Read the model definition and answer for the solid it produces. Units are mm, in the model's axes. Coordinates: 2 decimals unless noted, no trailing zeros. Order: outer loops, then holes, each group sorted by start corner. A loop starts at its lowest first (then second) coordinate and runs counter-clockwise, first axis right, second up. Notation, with made-up numbers: (66.25, -12.5) -> (117.25, -12.5) arc R8 cw to (117.25, -2.5) -> close; hole circle Ø2 at (-31.75, 35). An arc over 180 degrees is marked (long way). Answer as a JSON object with one key per item and string values. Group by question number.
1) Given pin 1 (1.5 mm diameter, centred on x = -0.5, y = 1.5, fed in from -Z); pin 2 (0.8 mm diameter, centred on x = -8, y = 1, fed in from +Z); pin 3 (0.8 mm diameter, centred on y = 1.5, z = 8, fed in from +X), each flat-ended and moving along its own axis, determine where each tip first touches the part or whether it passes through.
2) Section C-C on y = 2.5 is taken. Determine the outline of the cut face in (x, z), and give its area (3 significant figures).
3) Section B-B on x = 0 is taken. Determine the outline of the cut face in (y, z), and give its area (3 significant figures).
4) Determine the mould class of faces 1 (the cylindrical face through (9.7, 1.48, 6.18)), 2 (the flat face through (-3, 1, -8)), 3 (the flat face through (-2, 0, 0)) for opening direction Z: released by +Z, released by -Z, zero draft, split by the parting line, or undercut.
5) Section D-D on z = 7.5 is taken. Determine the outline of the cut face in (x, y), and give its area (3 significant figures).
6) Consider L1, parallel to X at y = 0.85, z = 0; L2, parallel to X at y = 2.15, z = 2.5; L3, parallel to Z at x = 2.25, y = 2.2. Determine where each line is inside the solid, lowest interval first.
7) Section A-A on z = 0 is taken. Determine the outline of the cut face in (x, y), and give its area (3 significant figures).
from build123d import *

# Parameters (mm, degrees)
SKETCH5_R           = 11.5
BOSS_EXTRUDE2_DEPTH = 3
SKETCH3_W           = 6
SKETCH3_H           = 2.5
SKETCH3_W_2         = 2.5
SKETCH3_H_2         = 6
CUT_EXTRUDE1_DEPTH  = 3
SKETCH6_R           = 1.35
CUT_EXTRUDE2_DEPTH  = 3


with BuildPart() as part:
    # Sketch5 → Boss-Extrude2 (new body)
    with BuildSketch(Plane(origin=(0, 0, 0), x_dir=(1, 0, 0), z_dir=(0, 1, 0))):
        with Locations(Location((0, 0, 0), (0, 0, 270))):
            Circle(SKETCH5_R)
    extrude(amount=BOSS_EXTRUDE2_DEPTH)

    # Sketch3 → Cut-Extrude1 (cut)
    with BuildSketch(Plane(origin=(0, 0, 0), x_dir=(1, 0, 0), z_dir=(0, 1, 0))):
        with Locations((0, 7.75)):
            Rectangle(SKETCH3_W, SKETCH3_H)
        with Locations((7.75, 0)):
            Rectangle(SKETCH3_W_2, SKETCH3_H_2)
        with Locations((0, -7.75)):
            Rectangle(SKETCH3_W, SKETCH3_H)
        with Locations((-7.75, 0)):
            Rectangle(SKETCH3_W_2, SKETCH3_H_2)
    extrude(amount=CUT_EXTRUDE1_DEPTH, mode=Mode.SUBTRACT)

    # Sketch6 → Cut-Extrude2 (cut)
    with BuildSketch(Plane(origin=(0, 3, 0), x_dir=(1, 0, 0), z_dir=(0, 1, 0))):
        with Locations(Location((0, 0, 0), (0, 0, 270))):
            Circle(SKETCH6_R)
    extrude(amount=-CUT_EXTRUDE2_DEPTH, mode=Mode.SUBTRACT)


solid = part.part
Worked answers:
{
 "1": {"pin 1": "stops at z = -11.5", "pin 2": "stops at z = 8.63", "pin 3": "stops at x = 8.63"},
 "2": {"outline": "circle Ø23 at (0, 0); hole (-9, -3) -> (-6.5, -3) -> (-6.5, 3) -> (-9, 3) -> close; hole (-3, -9) -> (3, -9) -> (3, -6.5) -> (-3, -6.5) -> close; hole (-3, 6.5) -> (3, 6.5) -> (3, 9) -> (-3, 9) -> close; hole circle Ø2.7 at (0, 0); hole (6.5, -3) -> (9, -3) -> (9, 3) -> (6.5, 3) -> close", "area": "350 mm²"},
 "3": {"outline": "(0, -11.5) -> (3, -11.5) -> (3, -9) -> (0, -9) -> close; (0, -6.5) -> (3, -6.5) -> (3, -1.35) -> (0, -1.35) -> close; (0, 1.35) -> (3, 1.35) -> (3, 6.5) -> (0, 6.5) -> close; (0, 9) -> (3, 9) -> (3, 11.5) -> (0, 11.5) -> close", "area": "45.9 mm²"},
 "4": {"face 1": "split by the parting line", "face 2": "undercut", "face 3": "zero draft"},
 "5": {"outline": "(-8.72, 0) -> (-3, 0) -> (-3, 3) -> (-8.72, 3) -> close; (3, 0) -> (8.72, 0) -> (8.72, 3) -> (3, 3) -> close", "area": "34.3 mm²"},
 "6": {"L1": "x = -11.5 to -9, -6.5 to -1.35, 1.35 to 6.5, 9 to 11.5", "L2": "x = -11.22 to -9, -6.5 to 6.5, 9 to 11.22", "L3": "z = -11.28 to -9, -6.5 to 6.5, 9 to 11.28"},
 "7": {"outline": "(-11.5, 0) -> (-9, 0) -> (-9, 3) -> (-11.5, 3) -> close; (-6.5, 0) -> (-1.35, 0) -> (-1.35, 3) -> (-6.5, 3) -> close; (1.35, 0) -> (6.5, 0) -> (6.5, 3) -> (1.35, 3) -> close; (9, 0) -> (11.5, 0) -> (11.5, 3) -> (9, 3) -> close", "area": "45.9 mm²"}
}
